```python
from build123d import *

# Parameters (mm, degrees)
F1_DEPTH = 6.35
F2_R     = 5.08
F4_DEPTH = 25.4
F5_W     = 8.255
F5_H     = 6.35
F6_DEPTH = 4.99459


with BuildPart() as f1:
    # F0 (on Front) → F1 (new body)
    with BuildSketch(Plane.XZ):
        Polygon((0, 3.175), (0, 0), (17.78, 0), (20.955, 0), (20.955, 3.175), align=None)
        Polygon((20.955, 0), (17.78, 0), (17.78, -23.114), (17.78, -29.464), (20.955, -29.464), align=None)
        Polygon((17.78, -29.464), (17.78, -23.114), (14.605, -23.114), align=None)
    extrude(amount=F1_DEPTH)

    # F2
    f2_edges = [f1.edges().sort_by_distance(p)[0] for p in [
        (20.955, -3.175, 3.175),
    ]]
    fillet(f2_edges, radius=F2_R)

    # F3 (on face) → F4 (cut)
    with BuildSketch(Plane.XY.offset(3.175)):
        with BuildLine():
            ThreePointArc((4.1275, -3.175), (3.6625320151, -4.2975320151), (2.54, -4.7625))
            Line((2.54, -4.7625), (12.7, -4.7625))
            ThreePointArc((12.7, -4.7625), (11.1125, -3.175), (12.7, -1.5875))
            Line((12.7, -1.5875), (2.54, -1.5875))
            ThreePointArc((2.54, -1.5875), (3.6625320151, -2.0524679849), (4.1275, -3.175))
        make_face()
        with BuildLine():
            ThreePointArc((2.54, -1.5875), (0.9525, -3.175), (2.54, -4.7625))
            Line((2.54, -4.7625), (2.54, -1.5875))
        make_face()
        with BuildLine():
            Line((2.54, -1.5875), (2.54, -4.7625))
            ThreePointArc((2.54, -4.7625), (3.6625320151, -4.2975320151), (4.1275, -3.175))
            ThreePointArc((4.1275, -3.175), (3.6625320151, -2.0524679849), (2.54, -1.5875))
        make_face()
        with BuildLine():
            ThreePointArc((12.7, -1.5875), (11.1125, -3.175), (12.7, -4.7625))
            Line((12.7, -4.7625), (12.7, -1.5875))
        make_face()
        with BuildLine():
            Line((12.7, -1.5875), (12.7, -4.7625))
            ThreePointArc((12.7, -4.7625), (13.8225320151, -4.2975320151), (14.2875, -3.175))
            ThreePointArc((14.2875, -3.175), (13.8225320151, -2.0524679849), (12.7, -1.5875))
        make_face()
    extrude(amount=-F4_DEPTH, mode=Mode.SUBTRACT)

    # F5 (on face) → F6 (cut)
    with BuildSketch(Plane.XY.offset(3.175)):
        with Locations((4.1275, -3.175)):
            Rectangle(F5_W, F5_H)
    extrude(amount=-F6_DEPTH, mode=Mode.SUBTRACT)


solid = f1.part
```
Verification items for the finished model (mm, model axes). A direction names the side the tool comes from. Give positions to 0.01 mm unless a question says otherwise; leave off trailing zeros. Order: outer loops, then holes, each group sorted by start corner. A loop starts at its lowest first (then second) coordinate and runs counter-clockwise, first axis right, second up. Notation, with made-up numbers: M -15,68.25 L 34,68.25 A15 cw 34,89.25 Z; hole C -29.5,45.25 d1. An arc over 180 degrees is marked long. Return JSON: item names as keys, results as strings. Group by question number.
1) Go/stop test with flat-tipped pins: pin 1 Ø3.5 at (x, z) = (10.5, 2.5) entering from +Y; pin 2 Ø3 at (x, y) = (14.5, -3) entering from -Z; pin 3 Ø1.9 at (y, z) = (-3.5, -7) entering from -X. Record where each tip stops, or that it passes through.
2) Access from +Z, -Z, +X, -X, +Y, -Y to the whole of each face (thin tool, end or side, straight path). Record for faces 1 (the face through (16.17, -3.13, -26.24)), 2 (the face through (17.78, -3, -11)), 3 (the face through (11, -1.588, 2)).
3) Section check C-C on x = 15.5. Record the cut outline in (y, z) (3 decimals), and give its area (3 significant figures).
4) Section check D-D on z = -2.5. Record the cut outline in (x, y) (3 decimals).
5) Scan lines: line 1 (X direction, y = -4.75, z = -10) (3 decimals); line 2 (Z direction, x = 9, y = -5.75) (3 decimals); line 3 (Z direction, x = 14.75, y = -4.75) (3 decimals). Record each from-to range of solid material in increasing order.
6) Section check B-B on y = -5.5. Record the cut outline in (x, z) (3 decimals), and give its area (3 significant figures).
7) Mould release check, pull along Z, two halves, no side actions. Record for faces 4 (the face through (16, -3, -23.114)), 5 (the face through (14, -2, 3.175)), 6 (the face through (8.255, -6, 2)): pulls with the +Z half, pulls with the -Z half, needs draft (parallel to the pull), parting line crosses it, or undercut.
Answer block:
{
 "1": {"pin 1": "stops at y = 0", "pin 2": "stops at z = -25.9", "pin 3": "stops at x = 17.78"},
 "2": {"face 1": "-Z, -X, +Y, -Y", "face 2": "-X, +Y, -Y", "face 3": "+Z, -Z, -X"},
 "3": {"outline": "M -6.35,-24.904 L 0,-24.904 L 0,-23.114 L -6.35,-23.114 Z; M -6.35,0 L 0,0 L 0,3.175 L -6.35,3.175 Z", "area": "31.5 mm^2"},
 "4": {"outline": "M 17.78,-6.35 L 20.955,-6.35 L 20.955,0 L 17.78,0 Z"},
 "5": {"line 1": "x = 17.78 to 20.955", "line 2": "z = 0 to 3.175", "line 3": "z = -23.404 to -23.114, 0 to 3.175"},
 "6": {"outline": "M 8.255,0 L 17.78,0 L 17.78,-23.114 L 14.605,-23.114 L 17.78,-29.464 L 20.955,-29.464 L 20.955,-1.905 A5.08 ccw 15.875,3.175 L 8.255,3.175 Z", "area": "138 mm^2"},
 "7": {"face 4": "undercut", "face 5": "pulls with the +Z half", "face 6": "needs draft"}
}
